from build123d import *

# Parameters (mm, degrees)
F0_R     = 1.016
F0_W     = 50.8
F0_H     = 5.08
F1_DEPTH = 5.08
F2_W     = 5.08
F2_H     = 44.45
F3_DEPTH = 5.081
F4_DEPTH = 5.08


with BuildPart() as f1:
    # F0 (on Front) → F1 (new body)
    with BuildSketch(Plane.XZ):
        Polygon((0, 88.9), (0, 0), (119.7864, 0), (170.5864, 0), (262.22198, 0), (313.02198, 0), (404.67026, 0), (455.47026, 0), (547.10584, 0), (597.90584, 0), (717.69224, 0), (717.69224, 88.9), (597.90584, 88.9), (547.10584, 88.9), (455.47026, 88.9), (404.67026, 88.9), (313.02198, 88.9), (262.22198, 88.9), (170.5864, 88.9), (119.7864, 88.9), align=None)
        with Locations((57.9374, 44.45)):
            Circle(F0_R, mode=Mode.SUBTRACT)
        with Locations((659.75484, 44.45)):
            Circle(F0_R, mode=Mode.SUBTRACT)
        with Locations((145.1864, 91.44)):
            Rectangle(F0_W, F0_H)
        with Locations((145.1864, -2.54)):
            Rectangle(F0_W, F0_H)
        with Locations((287.62198, -2.54)):
            Rectangle(F0_W, F0_H)
        with Locations((287.62198, 91.44)):
            Rectangle(F0_W, F0_H)
        with Locations((430.07026, 91.44)):
            Rectangle(F0_W, F0_H)
        with Locations((430.07026, -2.54)):
            Rectangle(F0_W, F0_H)
        with Locations((572.50584, 91.44)):
            Rectangle(F0_W, F0_H)
        with Locations((572.50584, -2.54)):
            Rectangle(F0_W, F0_H)
    extrude(amount=F1_DEPTH)

    # F2 (on face) → F3 (cut, through all)
    with BuildSketch(Plane.XZ.offset(5.08)):
        with Locations((2.54, 66.675)):
            Rectangle(F2_W, F2_H)
    extrude(amount=-F3_DEPTH, mode=Mode.SUBTRACT)

    # F2 (on face) → F4 (join)
    with BuildSketch(Plane.XZ.offset(5.08)):
        with Locations((720.23224, 66.675)):
            Rectangle(F2_W, F2_H)
    extrude(amount=-F4_DEPTH)


solid = f1.part
Can you work these out from the model? Positions are in its coordinate system, mm. Coordinates: 2 decimals unless noted, no trailing zeros. Write each loop counter-clockwise with the first axis right and the second up, starting at its lowest first coordinate (ties: lowest second). Pieces come first, ordered by that corner, then holes. Notation, with made-up numbers: (79, 79.25) -> (138, 79.25) arc R16 cw to (138, 92.25) -> close; hole circle Ø1 at (53, 87.25). An arc over 180 degrees is marked (long way). Write each question's results on one line, items separated by ' | '. Start each with the question number.
Item 1: If we section it at A-A, the plane y = -1.35: Count the separate pieces of the cut face and the enclosed holes in it, and give its area (3 significant figures).
Item 2: If we section it at B-B, the plane x = 385.5: Write out the boundary of the cut face in (y, z), and give its area (3 significant figures).
Item 3: I'm going to push flat-ended pins straight in: P1, Ø1.5, axis at y = -3, z = 90.5, coming from the -X side; P2, Ø2.5, axis at y = -3, z = 76.5, coming from the -X side; P3, Ø1.5, axis at x = 493, y = -2.5, coming from the -Z side. Where does each tip first touch, or does it pass through?
Item 4: Please list where these lines run through material, in increasing order: probe 1 along X at (y, z) = (-0.8, 89); probe 2 along Z at (x, y) = (38, -1.6); probe 3 along X at (y, z) = (-1.3, 69).
Answer block:
1) separate pieces: 1 | enclosed holes: 2 | area: 65,900 mm²
2) outline: (-5.08, 0) -> (0, 0) -> (0, 88.9) -> (-5.08, 88.9) -> close | area: 452 mm²
3) P1: x = 119.79 | P2: x = 5.08 | P3: z = 0
4) probe 1: 119.79 to 170.59, 262.22 to 313.02, 404.67 to 455.47, 547.11 to 597.91 | probe 2: 0 to 88.9 | probe 3: 5.08 to 722.77
